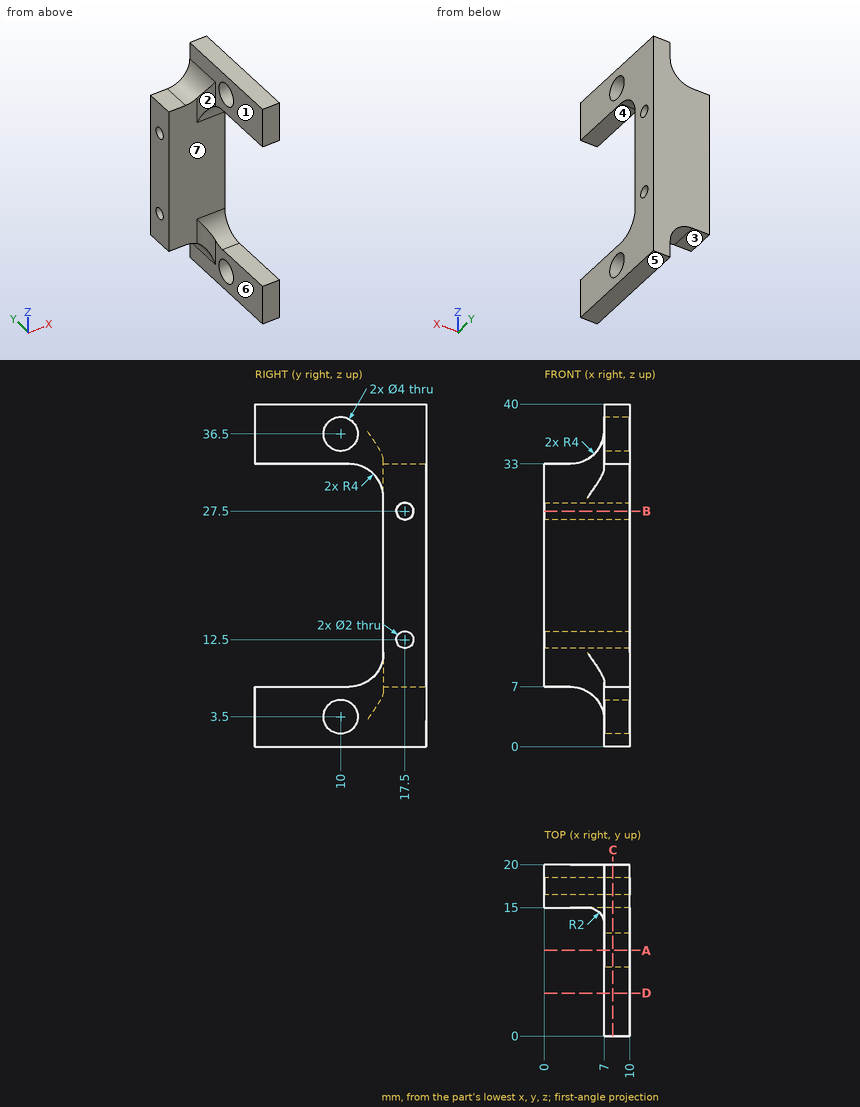
Design review of the part shown in the three views and the two pictorial views. Dimensions are in mm from the part's minimum x, y and z. A direction names the side the tool comes from. Round coordinates to 2 decimals unless told otherwise and drop trailing zeros. Write each loop counter-clockwise with the first axis right and the second up, starting at its lowest first coordinate (ties: lowest second). Pieces come first, ordered by that corner, then holes.
1) Machinability: for the marked faces 1, 2, 3 and 4, which of the approach directions +Z, -Z, +X, -X, +Y, -Y give a long, thin tool a straight path to every point of the face, cutting with its end or side? Answer none if there is none.
Answer below:
face 1: +Z, -X, -Y
face 2: +Z, -Z, -X, -Y
face 3: -Z, -X, +Y, -Y
face 4: +X, -X, -Y
2) Take a section at B-B on z = 27.5. Give the boundary of the cut face in (x, y).
Answer below:
outline: (0, 15) - (10, 15) - (10, 16.5) - (0, 16.5) - close; (0, 18.5) - (10, 18.5) - (10, 20) - (0, 20) - close
3) Take a section at C-C on x = 8. Give the boundary of the cut face in (y, z), then the cut area to 3 significant figures.
Answer below:
outline: (0, 0) - (20, 0) - (20, 40) - (0, 40) - (0, 33) - (11, 33) arc R4 cw to (15, 29) - (15, 11) arc R4 cw to (11, 7) - (0, 7) - close; hole circle Ø4 at (10, 3.5); hole circle Ø4 at (10, 36.5); hole circle Ø2 at (17.5, 12.5); hole circle Ø2 at (17.5, 27.5)
area: 385 mm2
4) Take a section at D-D on y = 5. Give the boundary of the cut face in (x, z).
Answer below:
outline: (7, 0) - (10, 0) - (10, 7) - (7, 7) - close; (7, 33) - (10, 33) - (10, 40) - (7, 40) - close
5) Mouldability with a two-part tool opening along Z and no side actions: class the marked faces 5, 6 and 7 as +Z half, -Z half, draft (parallel to the pull), parting line (faces both ways), or undercut.
Answer below:
face 5: -Z half
face 6: draft
face 7: undercut
6) Insertion check: pin 1 Ø1.5 at (x, y) = (8.5, 4.5) entering from -Z; pin 2 Ø4 at (x, z) = (3.5, 15) entering from -Y; pin 3 Ø1.5 at (x, y) = (1.5, 18.5) entering from +Z; pin 4 Ø6.5 at (y, z) = (10, 3.5) entering from -X. Each pin has a flat end and moves straight along its axis. Give the tip position at first contact, or say it passes through.
Answer below:
pin 1: stops at z = 0
pin 2: stops at y = 15
pin 3: stops at z = 33
pin 4: stops at x = 6.98
7) For line 1 along Y through (x, z) = (3, 12.5); line 2 along Y through (x, z) = (8.95, 3.5); line 3 along Z through (x, y) = (2, 17.75), list the stretches that pass through material, from the lowest coordinate up.
Answer below:
line 1: y = 15 to 16.5, 18.5 to 20
line 2: y = 0 to 8, 12 to 20
line 3: z = 7 to 11.53, 13.47 to 26.53, 28.47 to 33
8) Take a section at A-A on y = 10. Give the boundary of the cut face in (x, z).
Answer below:
outline: (7, 0) - (10, 0) - (10, 1.5) - (7, 1.5) - close; (7, 5.5) - (10, 5.5) - (10, 7) - (7, 7) - close; (7, 33) - (10, 33) - (10, 34.5) - (7, 34.5) - close; (7, 38.5) - (10, 38.5) - (10, 40) - (7, 40) - close
